Geometry: final body of the model. Coordinates: model frame, mm. Give positions to 0.01 mm unless a question says otherwise; leave off trailing zeros. Write each loop counter-clockwise with the first axis right and the second up, starting at its lowest first coordinate (ties: lowest second). Pieces come first, ordered by that corner, then holes.
Q1. Cut plane B-B on y = 42. Return the cut outline in (x, z), plus the area to 3 significant figures.
Q2. Line query: L1, parallel to Z at x = -1, y = 19; L2, parallel to Y at x = 12, z = 3.5; L3, parallel to Y at x = -26.5, z = 4.75. Output: solid intervals per line, ascending.
Q3. Cut plane A-A on x = -0.5. Return the cut outline in (y, z).
Q4. Pin query (flat end, axial travel): pin 1 (1.9 mm diameter, centred on y = 6.5, z = 4.5, fed in from -X); pin 2 (0.5 mm diameter, centred on x = 0.5, z = 5, fed in from -Y); pin 3 (1.5 mm diameter, centred on y = 8.5, z = 7, fed in from -X). Return the tip coordinate at first contact, or that it passes through.
```python
from build123d import *

# Parameters (mm, degrees)
F0_W     = 60
F0_H     = 110
F1_DEPTH = 8
F2_R     = 5
F3_R     = 5
F4_R     = 5
F5_DEPTH = 0.2
F6_R     = 5
F7_W     = 8.2122897729
F7_H     = 1.7597768456
F8_DEPTH = 0.8
F9_DEPTH = 25


with BuildPart() as f1:
    # F0 (on Top) → F1 (new body)
    with BuildSketch(Plane.XY):
        Rectangle(F0_W, F0_H)
    extrude(amount=F1_DEPTH)

    # F2
    f2_edges = [f1.edges().sort_by_distance(p)[0] for p in [
        (0, -55, 8),
    ]]
    fillet(f2_edges, radius=F2_R)

    # F3
    f3_edges = [f1.edges().sort_by_distance(p)[0] for p in [
        (30, 2.5, 8),
    ]]
    fillet(f3_edges, radius=F3_R)

    # F4
    f4_edges = [f1.edges().sort_by_distance(p)[0] for p in [
        (-2.5, 55, 8),
    ]]
    fillet(f4_edges, radius=F4_R)

    # F5 (add): a face of the model
    f5_faces = [f1.faces().sort_by_distance(p)[0] for p in [
        (30, 0, 1.5),
    ]]
    extrude(f5_faces, amount=F5_DEPTH)

    # F6
    f6_edges = [f1.edges().sort_by_distance(p)[0] for p in [
        (-30, 0, 8),
    ]]
    fillet(f6_edges, radius=F6_R)

    # F7 (on Front) → F8 (cut)
    with BuildSketch(Plane.XZ):
        with Locations((0, 4.8393858597)):
            Rectangle(F7_W, F7_H)
    extrude(amount=-F8_DEPTH, mode=Mode.SUBTRACT)

    # F7 (on Front) → F9 (cut)
    with BuildSketch(Plane.XZ):
        with Locations((0, 4.8393858597)):
            Rectangle(F7_W, F7_H)
    extrude(amount=-F9_DEPTH, mode=Mode.SUBTRACT)


solid = f1.part
```
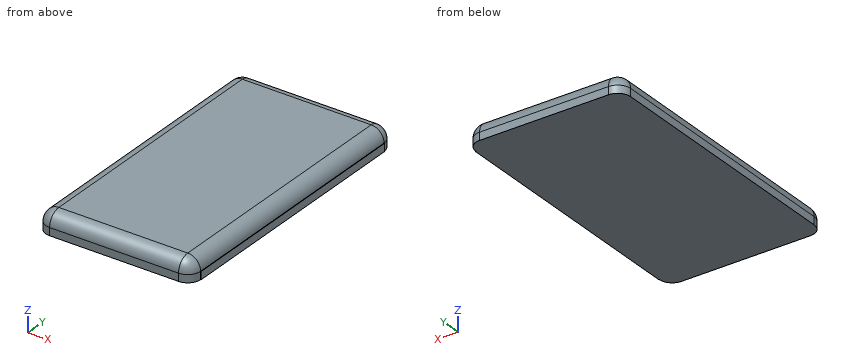
Data:
1. outline: (-30, 0) - (30.2, 0) - (30.2, 3) - (30, 3) arc R5 ccw to (25, 8) - (-25, 8) arc R5 ccw to (-30, 3) - close
1. area: 470 mm2
2. L1: z = 0 to 3.96, 5.72 to 8
2. L2: y = -54.97 to 54.97
2. L3: y = -54.44 to 54.44
3. outline: (-55, 0) - (55, 0) - (55, 3) arc R5 ccw to (50, 8) - (-50, 8) arc R5 ccw to (-55, 3) - close; hole (0, 3.96) - (25, 3.96) - (25, 5.72) - (0, 5.72) - close
4. pin 1: stops at x = -29.97
4. pin 2: stops at y = -54.68
4. pin 3: stops at x = -28.8
